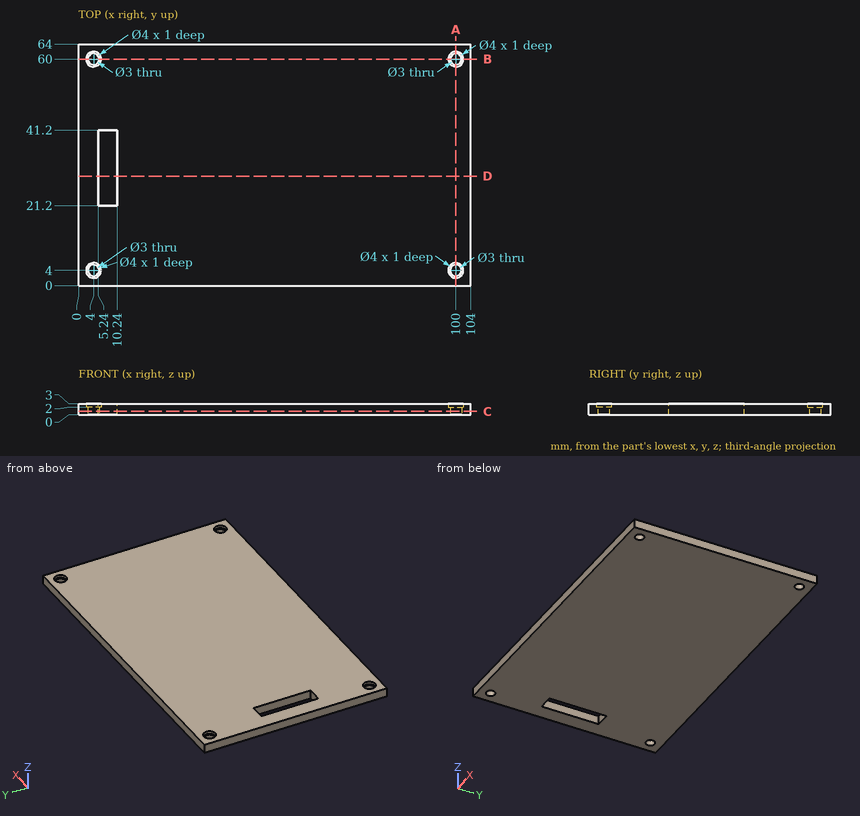
Answer from the drawing. Dimensions are ordinates in mm from the lowest x, y and z of the part. Coordinates: 2 decimals unless noted, no trailing zeros. Loops run counter-clockwise (first coordinate to the right, second up) from the corner with the lowest first, then second, coordinate; pieces in that order, holes last. Notation, with made-up numbers: (58.25, -27.5) - (85.25, -27.5) arc R15 cw to (85.25, -6.5) - close; hole circle Ø6 at (32, -11.5). An arc over 180 degrees is marked (long way). Answer in a Markdown table with one row per item.
1. Straight lines are drawn through the part: line 1 (Y direction, x = 4, z = 1.35); line 2 (Y direction, x = 100, z = 2.35); line 3 (X direction, y = 35, z = 1.1). For each, find the intervals that lie inside material, in ascending order.
Conclusion:
| item | result |
|---|---|
| line 1 | y = 0 to 2.5, 5.5 to 58.5, 61.5 to 64 |
| line 2 | y = 0 to 2, 6 to 58, 62 to 64 |
| line 3 | x = 0 to 5.24, 10.24 to 104 |
2. Find section B-B, the plane y = 60. Write down the section's boundary in (x, z).
Conclusion:
| item | result |
|---|---|
| outline | (0, 0) - (2.5, 0) - (2.5, 2) - (2, 2) - (2, 3) - (0, 3) - close; (5.5, 0) - (98.5, 0) - (98.5, 2) - (98, 2) - (98, 3) - (6, 3) - (6, 2) - (5.5, 2) - close; (101.5, 0) - (104, 0) - (104, 3) - (102, 3) - (102, 2) - (101.5, 2) - close |
3. Find section C-C, the plane z = 0.95. Write down the section's boundary in (x, y), then the cut area to 3 significant figures.
Conclusion:
| item | result |
|---|---|
| outline | (0, 0) - (104, 0) - (104, 64) - (0, 64) - close; hole circle Ø3 at (4, 4); hole circle Ø3 at (4, 60); hole (5.24, 21.2) - (10.24, 21.2) - (10.24, 41.2) - (5.24, 41.2) - close; hole circle Ø3 at (100, 4); hole circle Ø3 at (100, 60) |
| area | 6,530 mm² |
4. Find section D-D, the plane y = 29. Write down the section's boundary in (x, z).
Conclusion:
| item | result |
|---|---|
| outline | (0, 0) - (5.24, 0) - (5.24, 3) - (0, 3) - close; (10.24, 0) - (104, 0) - (104, 3) - (10.24, 3) - close |
5. Given pin 1 (2.5 mm diameter, centred on x = 100, y = 4, fed in from +Z); pin 2 (3.5 mm diameter, centred on x = 100, y = 60, fed in from +Z), each flat-ended and moving along its own axis, determine where each tip first touches the part or whether it passes through.
Conclusion:
| item | result |
|---|---|
| pin 1 | passes through |
| pin 2 | stops at z = 2 |
6. Find section A-A, the plane x = 100. Write down the section's boundary in (y, z).
Conclusion:
| item | result |
|---|---|
| outline | (0, 0) - (2.5, 0) - (2.5, 2) - (2, 2) - (2, 3) - (0, 3) - close; (5.5, 0) - (58.5, 0) - (58.5, 2) - (58, 2) - (58, 3) - (6, 3) - (6, 2) - (5.5, 2) - close; (61.5, 0) - (64, 0) - (64, 3) - (62, 3) - (62, 2) - (61.5, 2) - close |
